Autodesk Inventor part; units mm, degrees
ref_plane "YZ Plane" through (0, 0, 0) normal (1, 0, 0) x (0, 1, 0)
ref_plane "XZ Plane" through (0, 0, 0) normal (0, 1, 0) x (-1, 0, 0)
ref_plane "XY Plane" through (0, 0, 0) normal (0, 0, 1) x (1, 0, 0)
sketch "Sketch1" plane through (0, 0, 0) normal (0, 1, 0) x (-1, 0, 0)
  line L0 (-9.525, -9.525) -> (9.525, -9.525)
  line L1 (9.525, -9.525) -> (9.525, 9.525)
  line L2 (9.525, 9.525) -> (-9.525, 9.525)
  line L3 (-9.525, 9.525) -> (-9.525, -9.525)
  line L4 (-9.525, -9.525) -> (9.525, 9.525) construction
  line L5 (9.525, -9.525) -> (-9.525, 9.525) construction
  circle A0 centre (0, 0) radius 2.5527
  dimension "d0" = 19.05
  dimension "d1" = 19.05
  dimension "d2" = 5.1054
extrude "Extrusion1" add sketch "Sketch1" along normal blind 19.05
thread "Thread1"
properties part number "STRU_024_BilletBlock2" material "Aluminum 6061"
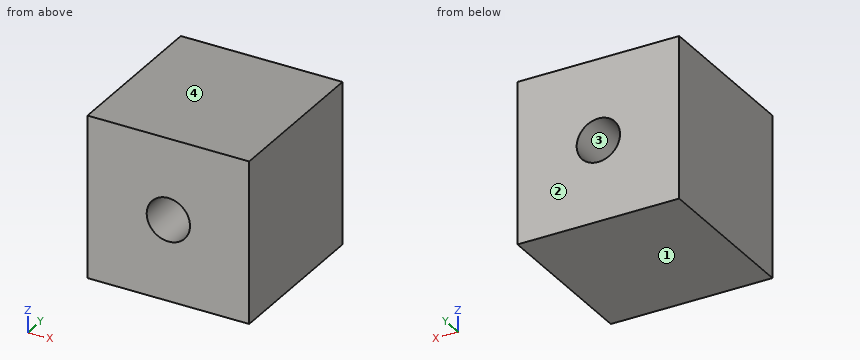
Check sheet for the modelled part. Datum: model origin and axes. Units: mm. Face numbers are marked on the shaded views. Coordinates: 2 decimals unless noted, no trailing zeros. Write each loop counter-clockwise with the first axis right and the second up, starting at its lowest first coordinate (ties: lowest second). Pieces come first, ordered by that corner, then holes. Notation, with made-up numbers: M 88.25,87.25 L 117.25,87.25 A26 ccw 117.25,101.25 Z; hole C 45.5,79 d8. An arc over 180 degrees is marked long. Answer as CSV lines item,"result".
Q1. Go/stop test with a flat-tipped pin: pin 1 (5 mm diameter, centred on x = 6.5, z = -4.5, fed in from -Y). Record where the tip stops, or that it passes through.
Check result:
pin 1,"y = 0"
Q2. Cross-section at C-C (y = 14.25). Record the boundary of the cut face in (x, z) (3 decimals), then the cut area to 3 significant figures.
Check result:
outline,"M -9.525,-9.525 L 9.525,-9.525 L 9.525,9.525 L -9.525,9.525 Z; hole C 0,0 d5.105"
area,"342 mm^2"
Q3. Mould release check, pull along Z, two halves, no side actions. Record for the marked faces 1, 2, 3 and 4: released by +Z, released by -Z, zero draft, split by the parting line, or undercut.
Check result:
face 1,"released by -Z"
face 2,"zero draft"
face 3,"undercut"
face 4,"released by +Z"
Q4. Cross-section at B-B (z = 0). Record the boundary of the cut face in (x, y) (3 decimals).
Check result:
outline,"M -9.525,0 L -2.553,0 L -2.553,19.05 L -9.525,19.05 Z; M 2.553,0 L 9.525,0 L 9.525,19.05 L 2.553,19.05 Z"
Q5. Cross-section at A-A (x = 0). Record the boundary of the cut face in (y, z) (3 decimals).
Check result:
outline,"M 0,-9.525 L 19.05,-9.525 L 19.05,-2.553 L 0,-2.553 Z; M 0,2.553 L 19.05,2.553 L 19.05,9.525 L 0,9.525 Z"
Q6. Material ranges on probe 1 along Z at (x, y) = (0, 4) (3 decimals); probe 2 along X at (y, z) = (14, 1.25) (3 decimals); probe 3 along Z at (x, y) = (1.5, 6.25) (1 decimal), recorded low to high. Write a range as from..to.
Check result:
probe 1,"-9.525..-2.553, 2.553..9.525"
probe 2,"-9.525..-2.226, 2.226..9.525"
probe 3,"-9.5..-2.1, 2.1..9.5"
